```python
from build123d import *

# Parameters (mm, degrees)
SKETCH_1_R          = 9
SKETCH_1_R_2        = 2.5
EXTRUDE_1_DEPTH     = 6
SKETCH_2_R          = 4.25
EXTRUDE_2_DEPTH     = 18
SKETCH_3_R          = 9
CUT_EXTRUDE_1_DEPTH = 26.740289584
SKETCH_4_R          = 9
CUT_EXTRUDE_2_DEPTH = 26.740289584
EXTRUDE_3_DEPTH     = 4
SKETCH_6_R          = 2.5
CUT_EXTRUDE_3_DEPTH = 15


with BuildPart() as part:
    # 草图1 → 凸台-拉伸1 (new body)
    with BuildSketch(Plane(origin=(0, 0, 0), x_dir=(1, 0, 0), z_dir=(0, 1, 0))):
        with Locations(Location((0, 0, 0), (0, 0, 270))):
            Circle(SKETCH_1_R)
        with Locations(Location((0, 0, 0), (0, 0, 270))):
            Circle(SKETCH_1_R_2, mode=Mode.SUBTRACT)
    extrude(amount=EXTRUDE_1_DEPTH)

    # 草图2 → 凸台-拉伸2 (add)
    with BuildSketch(Plane.XY.offset(23)):
        with Locations((0, 3)):
            Circle(SKETCH_2_R)
    extrude(amount=-EXTRUDE_2_DEPTH)

    # 草图3 → 切除-拉伸1 (cut, through all)
    with BuildSketch(Plane(origin=(0, 6, 0), x_dir=(1, 0, 0), z_dir=(0, 1, 0))):
        Circle(SKETCH_3_R)
    extrude(amount=CUT_EXTRUDE_1_DEPTH, mode=Mode.SUBTRACT)

    # 草图4 → 切除-拉伸2 (cut, through all)
    with BuildSketch(Plane.XZ):
        Circle(SKETCH_4_R)
    extrude(amount=CUT_EXTRUDE_2_DEPTH, mode=Mode.SUBTRACT)

    # 草图5 → 凸台-拉伸3 (add)
    with BuildSketch(Plane.XY.offset(23)):
        Polygon((0, 8.5), (-4.763139721, 5.75), (-4.763139721, 0.25), (0, -2.5), (4.763139721, 0.25), (4.763139721, 5.75), align=None)
    extrude(amount=EXTRUDE_3_DEPTH)

    # 草图6 → 切除-拉伸3 (cut)
    with BuildSketch(Plane.XY.offset(27)):
        with Locations((0, 3)):
            Circle(SKETCH_6_R)
    extrude(amount=-CUT_EXTRUDE_3_DEPTH, mode=Mode.SUBTRACT)


solid = part.part
```
Geometry: final body of the model. Coordinates: model frame, mm. A direction names the side the tool comes from. Round coordinates to 2 decimals unless told otherwise and drop trailing zeros. Order: outer loops, then holes, each group sorted by start corner. A loop starts at its lowest first (then second) coordinate and runs counter-clockwise, first axis right, second up. Notation, with made-up numbers: (22.25, 52.25) - (75.25, 52.25) arc R18 cw to (75.25, 76.25) - close; hole circle Ø3 at (64.5, -10). An arc over 180 degrees is marked (long way). Use CSV: the item, a comma, the result in double quotes. Start each with the question number.
Q1. First-contact query: pin 1 (4.5 mm diameter, centred on y = 3.5, z = 25, fed in from +X); pin 2 (1.2 mm diameter, centred on y = 4, z = 24.5, fed in from -X); pin 3 (5 mm diameter, centred on y = 5, z = 11.5, fed in from -X); pin 4 (2 mm diameter, centred on x = 7, z = 21.5, fed in from -Y). Flat tips, straight axial feed; report the tip coordinate or a pass-through.
Q2. Section query C-C (z = 19.5). Return loops of the section in (x, y).
Q3. Section query B-B (y = 2.5). Return loops of the section in (x, z).
Q4. Mould query, pull axis Z, two halves, no side actions, for faces 4 (the face through (2.348, -1.144, 24.972)), 5 (the face through (-2.44, 2.96, -0.54)), 6 (the face through (0, 6, 27)). Classes: +Z half, -Z half, draft (parallel to the pull), parting line (faces both ways), or undercut.
Q5. Section query A-A (z = 0). Return loops of the section in (x, y), and give its area (3 significant figures).
Q6. Material intervals for line 1 along Y through (x, z) = (0, 20); line 2 along Y through (x, z) = (-2.25, 8); line 3 along X through (y, z) = (2.25, 17), sorted ascending. Write a range as from..to.
Q7. Access query for faces 1 (the face through (0, 3, 12)), 2 (the face through (4.763, 3, 25)), 3 (the face through (-4, 1, 23)). Directions: +Z, -Z, +X, -X, +Y, -Y. A direction counts if a zero-diameter tool reaches every point of the face in a straight line with its end or side. Return the directions, or none.
Q8. Section query D-D (x = -7.75). Return loops of the section in (y, z).
Result set:
1,pin 1,"stops at x = 4.76"
1,pin 2,"stops at x = -4.76"
1,pin 3,"stops at x = -4.25"
1,pin 4,"passes through"
2,outline,"circle Ø8.5 at (0, 3); hole circle Ø5 at (0, 3)"
3,outline,"(-4.76, 23) - (-4.22, 23) - (-4.22, 7.95) arc R9 ccw (long way) to (4.22, 7.95) - (4.22, 23) - (4.76, 23) - (4.76, 27) - (2.45, 27) - (2.45, 12) - (-2.45, 12) - (-2.45, 27) - (-4.76, 27) - close; hole circle Ø5 at (0, 0)"
4,face 4,"draft"
4,face 5,"undercut"
4,face 6,"+Z half"
5,outline,"(-9, 0) - (-2.5, 0) - (-2.5, 6) - (-9, 6) - close; (2.5, 0) - (9, 0) - (9, 6) - (2.5, 6) - close"
5,area,"78.0 mm2"
6,line 1,"y = -1.25..0.5, 5.5..7.25"
6,line 2,"y = 0..6"
6,line 3,"x = -4.18..-2.38, 2.38..4.18"
7,face 1,"+Z"
7,face 2,"+Z, +X, +Y, -Y"
7,face 3,"none"
8,outline,"(0, -4.58) - (6, -4.58) - (6, 4.58) - (0, 4.58) - close"
